```python
from build123d import *

# Parameters (mm, degrees)
SKETCH1_W           = 80
SKETCH1_H           = 60
SKETCH1_R           = 24.25
BOSS_EXTRUDE1_DEPTH = 20
BOSS_EXTRUDE3_DEPTH = 15
SKETCH5_R           = 2.1
CUT_EXTRUDE2_DEPTH  = 10
SKETCH6_W           = 80
SKETCH6_H           = 20
BOSS_EXTRUDE4_DEPTH = 2
BOSS_EXTRUDE6_DEPTH = 50
SKETCH9_R           = 2.1
CUT_EXTRUDE3_DEPTH  = 100.619275243
SKETCH12_W          = 80
SKETCH12_H          = 70
SKETCH12_R          = 1.65
BOSS_EXTRUDE8_DEPTH = 8
BOSS_EXTRUDE9_DEPTH = 15
CUT_EXTRUDE4_START  = -10
SKETCH14_R          = 2.1
CUT_EXTRUDE4_DEPTH  = 10
SKETCH16_R          = 2
CUT_EXTRUDE5_DEPTH  = 3
CIRPATTERN1_COUNT   = 3


with BuildPart() as part:
    # Sketch1 → Boss-Extrude1 (new body)
    with BuildSketch(Plane.XY):
        Rectangle(SKETCH1_W, SKETCH1_H)
        Circle(SKETCH1_R, mode=Mode.SUBTRACT)
    extrude(amount=BOSS_EXTRUDE1_DEPTH)

    # Sketch4 → Boss-Extrude3 (add)
    with BuildSketch(Plane(origin=(40, 0, 0), x_dir=(0, 0, -1), z_dir=(1, 0, 0))):
        Polygon((-20, 30), (0, 30), (20, 30), (20, 20), (0, 20), (-20, 20), align=None)
    boss_extrude3 = extrude(amount=BOSS_EXTRUDE3_DEPTH)

    # Sketch5 → Cut-Extrude2 (cut)
    with BuildSketch(Plane(origin=(0, 30, 0), x_dir=(1, 0, 0), z_dir=(0, 1, 0))):
        with Locations(Location((47.5, -10, 0), (0, 0, 270))):
            Circle(SKETCH5_R)
        with Locations(Location((47.5, 10, 0), (0, 0, 270))):
            Circle(SKETCH5_R)
        Polygon((46, -20), (55, -15), (55, -20), align=None)
    cut_extrude2 = extrude(amount=-CUT_EXTRUDE2_DEPTH, mode=Mode.SUBTRACT)

    # Sketch6 → Boss-Extrude4 (add)
    with BuildSketch(Plane(origin=(0, -30, 0), x_dir=(-1, 0, 0), z_dir=(0, -1, 0))):
        with Locations((0, -10)):
            Rectangle(SKETCH6_W, SKETCH6_H)
    boss_extrude4 = extrude(amount=BOSS_EXTRUDE4_DEPTH)

    # Sketch8 → Boss-Extrude6 (add)
    with BuildSketch(Plane(origin=(0, 0, 0), x_dir=(-1, 0, 0), z_dir=(0, 0, -1))):
        Polygon((-40, -11), (-19, -32), (-40, -32), align=None)
    boss_extrude6 = extrude(amount=BOSS_EXTRUDE6_DEPTH)

    # Sketch9 → Cut-Extrude3 (cut, through all)
    with BuildSketch(Plane(origin=(40, 0, 0), x_dir=(0, 0, -1), z_dir=(1, 0, 0))):
        with Locations((27, -28)):
            Circle(SKETCH9_R)
    cut_extrude3 = extrude(amount=-CUT_EXTRUDE3_DEPTH, mode=Mode.SUBTRACT)

    # Sketch12 → Boss-Extrude8 (add)
    with BuildSketch(Plane.XZ.offset(32)):
        with Locations((0, -15)):
            Rectangle(SKETCH12_W, SKETCH12_H)
        with Locations(Location((-8, -8.3, 0), (0, 0, 270))):
            Circle(SKETCH12_R, mode=Mode.SUBTRACT)
        with Locations(Location((8, -8.3, 0), (0, 0, 270))):
            Circle(SKETCH12_R, mode=Mode.SUBTRACT)
        with Locations(Location((8, -38.3, 0), (0, 0, 270))):
            Circle(SKETCH12_R, mode=Mode.SUBTRACT)
        with Locations(Location((-8, -38.3, 0), (0, 0, 270))):
            Circle(SKETCH12_R, mode=Mode.SUBTRACT)
    extrude(amount=BOSS_EXTRUDE8_DEPTH)

    # Mirror1: Boss-Extrude3, Cut-Extrude2, Boss-Extrude4, Boss-Extrude6, Cut-Extrude3 across plane
    add(boss_extrude3.mirror(Plane(origin=(0, 0, 0), x_dir=(0, 0, 1), z_dir=(1, 0, 0))))
    add(cut_extrude2.mirror(Plane(origin=(0, 0, 0), x_dir=(0, 0, 1), z_dir=(1, 0, 0))), mode=Mode.SUBTRACT)
    add(boss_extrude4.mirror(Plane(origin=(0, 0, 0), x_dir=(0, 0, 1), z_dir=(1, 0, 0))))
    add(boss_extrude6.mirror(Plane(origin=(0, 0, 0), x_dir=(0, 0, 1), z_dir=(1, 0, 0))))
    add(cut_extrude3.mirror(Plane(origin=(0, 0, 0), x_dir=(0, 0, 1), z_dir=(1, 0, 0))), mode=Mode.SUBTRACT)

    # Sketch13 → Boss-Extrude9 (add)
    with BuildSketch(Plane.ZY.offset(40)):
        Polygon((20, -40), (0, -40), (-20, -40), (-20, -32), (0, -32), (20, -32), align=None)
    boss_extrude9 = extrude(amount=BOSS_EXTRUDE9_DEPTH)

    # Sketch14 → Cut-Extrude4 (cut)
    with BuildSketch(Plane.XZ.offset(40).offset(CUT_EXTRUDE4_START)):
        with Locations(Location((-47.5, 10, 0), (0, 0, 90))):
            Circle(SKETCH14_R)
        with Locations(Location((-47.5, -10, 0), (0, 0, 90))):
            Circle(SKETCH14_R)
    cut_extrude4 = extrude(amount=CUT_EXTRUDE4_DEPTH, mode=Mode.SUBTRACT)

    # Mirror2: Boss-Extrude9, Cut-Extrude4 across plane
    add(boss_extrude9.mirror(Plane(origin=(0, 0, 0), x_dir=(0, 0, 1), z_dir=(1, 0, 0))))
    add(cut_extrude4.mirror(Plane(origin=(0, 0, 0), x_dir=(0, 0, 1), z_dir=(1, 0, 0))), mode=Mode.SUBTRACT)

    # Sketch16 → Cut-Extrude5 (cut)
    with BuildSketch(Plane.XY.offset(20)):
        with Locations((0, -30)):
            Circle(SKETCH16_R)
    cut_extrude5 = extrude(amount=-CUT_EXTRUDE5_DEPTH, mode=Mode.SUBTRACT)

    # CirPattern1: Cut-Extrude5 ×3 about axis
    cirpattern1_axis = Axis((0, 0, 0), (0, 0, 1))
    for i in range(1, CIRPATTERN1_COUNT):
        add(cut_extrude5.rotate(cirpattern1_axis, i * 360 / CIRPATTERN1_COUNT), mode=Mode.SUBTRACT)


solid = part.part
```
The model under review builds one solid part; all positions refer to its coordinate system, in mm. A direction names the side the tool comes from. Give positions to 0.01 mm unless a question says otherwise; leave off trailing zeros. Write each loop counter-clockwise with the first axis right and the second up, starting at its lowest first coordinate (ties: lowest second). Pieces come first, ordered by that corner, then holes.
(1) Consider section C-C, the plane x = 32. Give the boundary of the cut face in (y, z), and give its area (3 significant figures).
(2) The part is to be moulded in two halves that separate along X. For faces 1 (the cylindrical face through (-45.45, 25.07, -10.46)), 2 (the flat face through (-47, 20, 0)), 3 (the flat face through (50.437, 25.07, 17.535)), say which applies: released by +X, released by -X, zero draft, split by the parting line, or undercut.
(3) For P1, Ø5, axis at x = 47.5, z = 10, coming from the +Y side; P2, Ø4, axis at x = 39, z = -38, coming from the +Y side; P3, Ø3.5, axis at x = -47.5, z = -10, coming from the -Y side; P4, Ø3, axis at x = -25.98, y = 15, coming from the -Z side, all flat-tipped, find the tip position at first contact; note any pin that passes through.
(4) Tool access review of faces 4 (the flat face through (47, -36, -20)), 5 (the flat face through (-55, -36, 0)), 6 (the flat face through (26, 15, 17)), 7 (the cylindrical face through (45.45, -35.94, -10.46)), 8 (the flat face through (47, -32, 0)): name each direction out of +Z, -Z, +X, -X, +Y, -Y from which nothing blocks a thin tool from reaching the whole face with its end or side.
(5) To check wall thickness, follow L1, parallel to Y at x = 0, z = 19; L2, parallel to X at y = 26, z = -10; L3, parallel to Y at x = 45.5, z = 7.5. State the ranges of each line that lie inside material, in increasing order.
(6) Consider section B-B, the plane y = 0. Give the boundary of the cut face in (x, z).
(7) Consider section D-D, the plane x = 8. Give the boundary of the cut face in (y, z).
(8) Consider section A-A, the plane z = 10. Give the number of separate pieces and of enclosed holes in the cut face, and give its area (3 significant figures).
Returned:
1. outline: (-40, -50) - (-19, -50) - (-19, 0) - (30, 0) - (30, 20) - (-40, 20) - close; hole circle Ø4.2 at (-28, -27)
1. area: 2,440 mm2
2. face 1: undercut
2. face 2: zero draft
2. face 3: released by +X
3. P1: stops at y = 30
3. P2: stops at y = -11
3. P3: passes through
3. P4: stops at z = 0
4. face 4: -Z, +X, +Y, -Y
4. face 5: +Z, -Z, -X, +Y, -Y
4. face 6: +Z
4. face 7: +Y, -Y
4. face 8: +Z, -Z, +X
5. L1: y = -40 to -32, -28 to -24.25, 24.25 to 30
5. L2: x = -55 to -49.6, -45.4 to -40, 40 to 45.4, 49.6 to 55
5. L3: y = -40 to -32, 20 to 30
6. outline: (-40, 0) - (-24.25, 0) - (-24.25, 20) - (-40, 20) - close; (24.25, 0) - (40, 0) - (40, 20) - (24.25, 20) - close
7. outline: (-40, -50) - (-32, -50) - (-32, -39.95) - (-40, -39.95) - close; (-40, -36.65) - (-32, -36.65) - (-32, -9.95) - (-40, -9.95) - close; (-40, -6.65) - (-32, -6.65) - (-32, 0) - (-22.89, 0) - (-22.89, 20) - (-40, 20) - close; (22.89, 0) - (30, 0) - (30, 20) - (22.89, 20) - close
8. separate pieces: 5
8. enclosed holes: 1
8. area: 4,140 mm2
